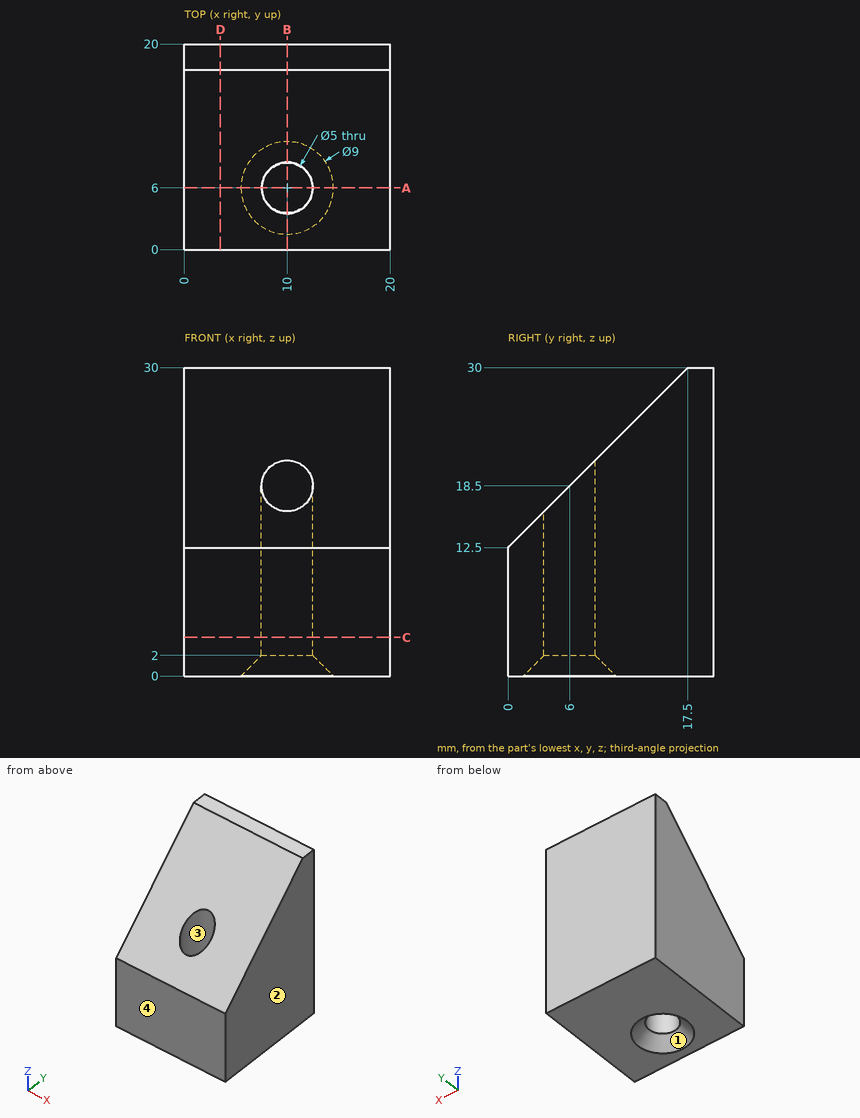
Verification items for this drawing (mm, ordinates from the low corner). Round coordinates to 2 decimals unless told otherwise and drop trailing zeros. Write each loop counter-clockwise with the first axis right and the second up, starting at its lowest first coordinate (ties: lowest second). Pieces come first, ordered by that corner, then holes. Notation, with made-up numbers: (15.25, 73) - (45.25, 73) arc R9 ccw to (45.25, 79) - close; hole circle Ø4 at (54.5, -20.75). An arc over 180 degrees is marked (long way). Answer as a JSON object with one key per item and string values. Group by question number.
Q1. Mould release check, pull along X, two halves, no side actions. Record for the marked faces 1, 2, 3 and 4: released by +X, released by -X, zero draft, split by the parting line, or undercut.
Q2. Go/stop test with flat-tipped pins: pin 1 Ø8 at (x, y) = (7, 16.5) entering from +Z; pin 2 Ø10 at (x, z) = (10.5, 19.5) entering from -Y; pin 3 Ø8 at (x, y) = (10, 6) entering from +Z. Record where each tip stops, or that it passes through.
Q3. Thickness scan on line 1 (Y direction, x = 10, z = 10.5); line 2 (Y direction, x = 9.5, z = 11); line 3 (Z direction, x = 13.25, y = 14). Record the ranges inside material, lowest first.
Q4. Section check A-A, the plane y = 6. Enter the section's corners in (x, z).
Q5. Section check B-B, the plane x = 10. Enter the section's corners in (y, z), plus the area to 3 significant figures.
Q6. Section check D-D, the plane x = 3.5. Enter the section's corners in (y, z), plus the area to 3 significant figures.
Q7. Section check C-C, the plane z = 3.75. Enter the section's corners in (x, y), plus the area to 3 significant figures.
Found:
{
 "1": {"face 1": "undercut", "face 2": "released by +X", "face 3": "undercut", "face 4": "zero draft"},
 "2": {"pin 1": "stops at z = 30", "pin 2": "stops at y = 2", "pin 3": "stops at z = 22.5"},
 "3": {"line 1": "y = 0 to 3.5, 8.5 to 20", "line 2": "y = 0 to 3.55, 8.45 to 20", "line 3": "z = 0 to 26.5"},
 "4": {"outline": "(0, 0) - (5.5, 0) - (7.5, 2) - (7.5, 18.5) - (0, 18.5) - close; (12.5, 2) - (14.5, 0) - (20, 0) - (20, 18.5) - (12.5, 18.5) - close"},
 "5": {"outline": "(0, 0) - (1.5, 0) - (3.5, 2) - (3.5, 16) - (0, 12.5) - close; (8.5, 2) - (10.5, 0) - (20, 0) - (20, 30) - (17.5, 30) - (8.5, 21) - close", "area": "350 mm^2"},
 "6": {"outline": "(0, 0) - (20, 0) - (20, 30) - (17.5, 30) - (0, 12.5) - close", "area": "447 mm^2"},
 "7": {"outline": "(0, 0) - (20, 0) - (20, 20) - (0, 20) - close; hole circle Ø5 at (10, 6)", "area": "380 mm^2"}
}
